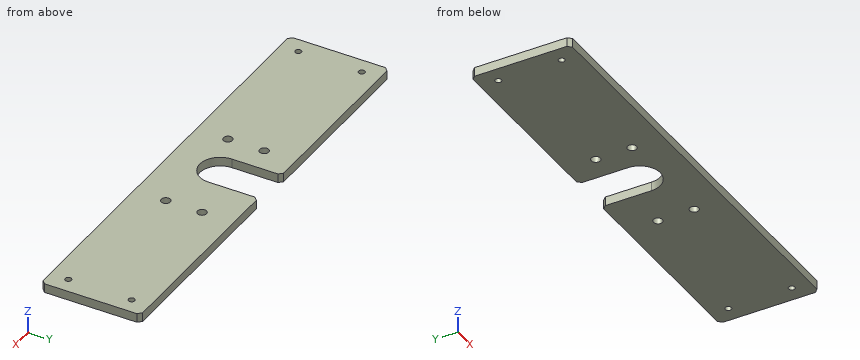
```python
from build123d import *

# Parameters (mm, degrees)
F0_R     = 6.35
F1_DEPTH = 12.7
F2_SIZE  = 5.08
F3_R     = 4.3561
F4_DEPTH = 12.701


with BuildPart() as f1:
    # F0 (on Top) → F1 (new body)
    with BuildSketch(Plane.XY):
        with BuildLine():
            Line((0, 139.7), (0, 0))
            Line((0, 0), (609.6, 0))
            Line((609.6, 0), (609.6, 139.7))
            Line((609.6, 139.7), (333.375, 139.7))
            Line((333.375, 139.7), (320.675, 139.7))
            Line((320.675, 139.7), (320.675, 69.85))
            ThreePointArc((320.675, 69.85), (292.1, 41.275), (263.525, 69.85))
            Line((263.525, 69.85), (263.525, 139.7))
            Line((263.525, 139.7), (0, 139.7))
        make_face()
        with Locations((228.6, 44.45)):
            Circle(F0_R, mode=Mode.SUBTRACT)
        with Locations((381, 44.45)):
            Circle(F0_R, mode=Mode.SUBTRACT)
        with Locations((228.6, 95.25)):
            Circle(F0_R, mode=Mode.SUBTRACT)
        with Locations((381, 95.25)):
            Circle(F0_R, mode=Mode.SUBTRACT)
    extrude(amount=F1_DEPTH)

    # F2
    f2_edges = [f1.edges().sort_by_distance(p)[0] for p in [
        (320.675, 139.7, 6.35),
        (0, 0, 6.35),
        (0, 139.7, 6.35),
        (263.525, 139.7, 6.35),
        (609.6, 139.7, 6.35),
        (609.6, 0, 6.35),
    ]]
    chamfer(f2_edges, length=F2_SIZE)

    # F3 (on face) → F4 (cut, through all)
    with BuildSketch(Plane.XY.offset(12.7)):
        with Locations((22.606, 114.3)):
            Circle(F3_R)
        with Locations((22.606, 25.4)):
            Circle(F3_R)
        with Locations((586.994, 25.4)):
            Circle(F3_R)
        with Locations((586.994, 114.3)):
            Circle(F3_R)
    extrude(amount=-F4_DEPTH, mode=Mode.SUBTRACT)


solid = f1.part
```
CAD build for the part. Positions are in the model's coordinates, mm. Coordinates: 2 decimals unless noted, no trailing zeros. Loops run counter-clockwise (first coordinate to the right, second up) from the corner with the lowest first, then second, coordinate; pieces in that order, holes last. Notation, with made-up numbers: (69.25, -0.75) - (99.25, -0.75) arc R34 ccw to (99.25, 30.25) - close; hole circle Ø5 at (88, 26). An arc over 180 degrees is marked (long way). Return JSON: item names as keys, results as strings.
1. Band-saw the part on B-B (z = 9). State how many separate pieces and enclosed holes the cut face has, and give its area (3 significant figures).
Result:
{"separate pieces": "1", "enclosed holes": "8", "area": "79,100 mm2"}
2. Probe L1, parallel to Y at x = 228.6, z = 9; L2, parallel to Y at x = 385.5, z = 4.75; L3, parallel to X at y = 85, z = 4 (3 decimals). List the from-to ranges inside material, lowest first. Write a range as from..to.
Result:
{"L1": "y = 0..38.1, 50.8..88.9, 101.6..139.7", "L2": "y = 0..39.97, 48.93..90.77, 99.73..139.7", "L3": "x = 0..263.525, 320.675..609.6"}
3. Band-saw the part on D-D (x = 292.1). Give the cut face in (y, z) (3 decimals), and give its area (3 significant figures).
Result:
{"outline": "(0, 0) - (41.275, 0) - (41.275, 12.7) - (0, 12.7) - close", "area": "524 mm2"}
4. Band-saw the part on C-C (y = 95.25). Give the cut face in (x, z) (3 decimals).
Result:
{"outline": "(0, 0) - (222.25, 0) - (222.25, 12.7) - (0, 12.7) - close; (234.95, 0) - (263.525, 0) - (263.525, 12.7) - (234.95, 12.7) - close; (320.675, 0) - (374.65, 0) - (374.65, 12.7) - (320.675, 12.7) - close; (387.35, 0) - (609.6, 0) - (609.6, 12.7) - (387.35, 12.7) - close"}
5. Band-saw the part on A-A (x = 381). Give the cut face in (y, z).
Result:
{"outline": "(0, 0) - (38.1, 0) - (38.1, 12.7) - (0, 12.7) - close; (50.8, 0) - (88.9, 0) - (88.9, 12.7) - (50.8, 12.7) - close; (101.6, 0) - (139.7, 0) - (139.7, 12.7) - (101.6, 12.7) - close"}
6. Drop a flat-ended pin along its axis: pin 1 (14.5 mm diameter, centred on x = 228.6, y = 95.25, fed in from +Z). Give the stop position or say it passes through.
Result:
{"pin 1": "stops at z = 12.7"}
